Can you work these out from the model? Positions are in its coordinate system, mm. A direction names the side the tool comes from. Give positions to 0.01 mm unless a question says otherwise; leave off trailing zeros. Order: outer loops, then holes, each group sorted by start corner. A loop starts at its lowest first (then second) coordinate and runs counter-clockwise, first axis right, second up.
```python
from build123d import *

# Parameters (mm, degrees)
SKETCH_1_W          = 1800
SKETCH_1_H          = 250
EXTRUDE_1_DEPTH     = 170
SKETCH_4_W          = 78.5
SKETCH_4_H          = 224
CUT_EXTRUDE_4_DEPTH = 1826.212316417
FILLET_1_R          = 13
FILLET_2_R          = 13
FILLET_3_R          = 13
FILLET_4_R          = 13


with BuildPart() as part:
    # 草图1 → 拉伸1 (new body)
    with BuildSketch(Plane.XY):
        with Locations((900, 125)):
            Rectangle(SKETCH_1_W, SKETCH_1_H)
    extrude(amount=EXTRUDE_1_DEPTH)

    # 草图4 → 切除-拉伸4 (cut, through all)
    with BuildSketch(Plane.ZY):
        with Locations((39.25, 125)):
            Rectangle(SKETCH_4_W, SKETCH_4_H)
        with Locations((130.75, 125)):
            Rectangle(SKETCH_4_W, SKETCH_4_H)
    extrude(amount=-CUT_EXTRUDE_4_DEPTH, mode=Mode.SUBTRACT)

    # 圆角1
    fillet_1_edges = [part.edges().sort_by_distance(p)[0] for p in [
        (900, 13, 170),
    ]]
    fillet(fillet_1_edges, radius=FILLET_1_R - 0.0001)  # a hair under: the kernel refuses the full size

    # 圆角2
    fillet_2_edges = [part.edges().sort_by_distance(p)[0] for p in [
        (900, 13, 0),
    ]]
    fillet(fillet_2_edges, radius=FILLET_2_R - 0.0001)  # a hair under: the kernel refuses the full size

    # 圆角3
    fillet_3_edges = [part.edges().sort_by_distance(p)[0] for p in [
        (900, 237, 170),
    ]]
    fillet(fillet_3_edges, radius=FILLET_3_R - 0.0001)  # a hair under: the kernel refuses the full size

    # 圆角4
    fillet_4_edges = [part.edges().sort_by_distance(p)[0] for p in [
        (900, 237, 0),
    ]]
    fillet(fillet_4_edges, radius=FILLET_4_R - 0.0001)  # a hair under: the kernel refuses the full size


solid = part.part
```
1) If I drill on line 1 (Y direction, x = 219, z = 26); line 2 (Z direction, x = 435.5, y = 101); line 3 (Y direction, x = 992, z = 8), over which ranges is the centre line in solid material (lowest first)?
2) Suppose I cut it at C-C (y = 87). Please give me the cut outline in (x, z), and give its area (3 significant figures).
3) Which directions (+Z, -Z, +X, -X, +Y, -Y) give clear straight access to the entire face, cutting with the end or side of a thin tool? Please do faces 1 (the face through (887, 13, 45)), 2 (the face through (887, 237, 124)), 3 (the face through (0, 124, 85)).
4) We'd pull the mould along Y, two halves only. Please class faces 4 (the face through (887, 250, 84)), 5 (the face through (887, 123, 91.5)), 6 (the face through (887, 0, 84)), 7 (the face through (887, 237, 45)): +Y half, -Y half, draft (parallel to the pull), parting line (faces both ways), or undercut.
5) I'm going to push flat-ended pins straight in: pin 1 Ø8 at (x, y) = (1132.5, 67) entering from -Z; pin 2 Ø6 at (x, y) = (328, 177.5) entering from +Z. Where does each tip first touch, or does it pass through?
6) Suppose I cut it at B-B (z = 29.5). Please give me the cut outline in (x, y).
Results:
1. line 1: y = 0 to 13, 237 to 250
1. line 2: z = 78.5 to 91.5
1. line 3: y = 0 to 12, 238 to 250
2. outline: (0, 78.5) - (1800, 78.5) - (1800, 91.5) - (0, 91.5) - close
2. area: 23,400 mm2
3. face 1: -Z, +X, -X
3. face 2: +Z, +X, -X
3. face 3: +Z, -Z, -X, +Y, -Y
4. face 4: +Y half
4. face 5: undercut
4. face 6: -Y half
4. face 7: undercut
5. pin 1: stops at z = 78.5
5. pin 2: stops at z = 91.5
6. outline: (0, 0) - (1800, 0) - (1800, 13) - (0, 13) - close; (0, 237) - (1800, 237) - (1800, 250) - (0, 250) - close
